Can you work these out from the model? Positions are in its coordinate system, mm. Round coordinates to 2 decimals unless told otherwise and drop trailing zeros. Loops run counter-clockwise (first coordinate to the right, second up) from the corner with the lowest first, then second, coordinate; pieces in that order, holes last.
(1) I want a section at B-B on x = -22. Write out the boundary of the cut face in (y, z).
(2) I want a section at A-A on y = 3.05. Write out the boundary of the cut face in (x, z).
(3) Will this pin go through, and if not, where does the flat tip stop? pin 1 Ø2 at (x, z) = (12.5, 19) entering from +Y.
(4) If I drill on line 1 along Z through (x, y) = (-16, 4.25); line 2 along X through (y, z) = (2.15, 38); line 3 along Y through (x, z) = (14, 30.5), over which ranges is the centre line in solid material (lowest first)?
(5) I want a section at D-D on x = 6. Write out the boundary of the cut face in (y, z), plus the area to 3 significant figures.
(6) I want a section at C-C on z = 3. Write out the boundary of the cut face in (x, y), plus the area to 3 significant figures.
Autodesk Inventor part; units mm, degrees
ref_plane "YZ Plane" through (0, 0, 0) normal (1, 0, 0) x (0, 1, 0)
ref_plane "XZ Plane" through (0, 0, 0) normal (0, 1, 0) x (-1, 0, 0)
ref_plane "XY Plane" through (0, 0, 0) normal (0, 0, 1) x (1, 0, 0)
sketch "Эскиз1" plane through (0, 0, 0) normal (0, 1, 0) x (-1, 0, 0)
  line L0 (0, 0) -> (-25, 0)
  line L1 (-25, 0) -> (-25, 20)
  line L2 (-25, 20) -> (0, 20)
  line L3 (0, 20) -> (0, 0)
  dimension "d0" = 25
  dimension "d1" = 20
extrude "Выдавливание1" add sketch "Эскиз1" along normal blind 2
sketch "Эскиз2" plane through (0, 2, 0) normal (0, 1, 0) x (1, 0, 0)
  line L0 (25, -20) -> (25, 0)
  line L1 (25, 0) -> (10, 0)
  line L2 (10, 0) -> (10, -5)
  line L3 (10, -5) -> (25, -5)
  line L4 (25, -5) -> (25, 0)
  point P0 (0, 0)
  dimension "d4" = 15
  dimension "d5" = 5
extrude "Выдавливание2" add sketch "Эскиз2" along normal blind 4
mirror "Зеркальное отражение1" about plane through (0, 0, 20) normal (0, 0, 1)
mirror "Зеркальное отражение2" about plane through (0, 0, 0) normal (-1, 0, 0)
properties part number "крышка кожуха нижняя"
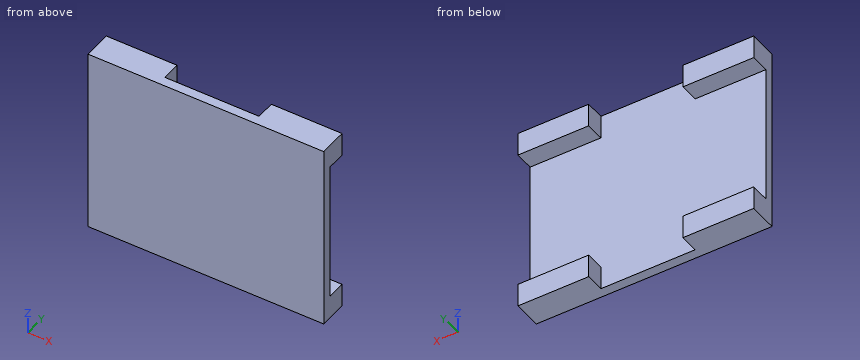
Filled sheet:
1. outline: (0, 0) - (6, 0) - (6, 5) - (2, 5) - (2, 35) - (6, 35) - (6, 40) - (0, 40) - close
2. outline: (-25, 0) - (-10, 0) - (-10, 5) - (-25, 5) - close; (-25, 35) - (-10, 35) - (-10, 40) - (-25, 40) - close; (10, 0) - (25, 0) - (25, 5) - (10, 5) - close; (10, 35) - (25, 35) - (25, 40) - (10, 40) - close
3. pin 1: stops at y = 2
4. line 1: z = 0 to 5, 35 to 40
4. line 2: x = -25 to -10, 10 to 25
4. line 3: y = 0 to 2
5. outline: (0, 0) - (2, 0) - (2, 40) - (0, 40) - close
5. area: 80.0 mm2
6. outline: (-25, 0) - (25, 0) - (25, 6) - (10, 6) - (10, 2) - (-10, 2) - (-10, 6) - (-25, 6) - close
6. area: 220 mm2
